```python
from build123d import *

# Parameters (mm, degrees)
BOSS_EXTRU_1_DEPTH      = 26
ESQUISSE2_R             = 12
ENL_V_MAT_EXTRU_1_DEPTH = 27
ESQUISSE3_W             = 35.8
ESQUISSE3_H             = 18
ESQUISSE3_W_2           = 20.2
ESQUISSE3_H_2           = 20.2
ENL_V_MAT_EXTRU_2_DEPTH = 43.5
ESQUISSE4_W             = 15
ESQUISSE4_H             = 20
ENL_V_MAT_EXTRU_3_DEPTH = 38.5
D_GAGEMENT_M31_D        = 3.3
ENL_V_MAT_EXTRU_4_REACH = 48.2
ESQUISSE7_W             = 6
ESQUISSE7_H             = 16
D_GAGEMENT_M41_D        = 4.4
D_GAGEMENT_M41_DEPTH    = 24
ESQUISSE10_W            = 2.2
ESQUISSE10_H            = 24
ENL_V_MAT_EXTRU_5_REACH = 5
ESQUISSE12_W            = 3
ESQUISSE12_H            = 7


with BuildPart() as part:
    # Esquisse1 → Boss.-Extru.1 (new body)
    with BuildSketch(Plane.XY):
        Polygon((0, 0), (0, -42.5), (86, -42.5), (86, -18.5), (71, 0), align=None)
    extrude(amount=BOSS_EXTRU_1_DEPTH)

    # Esquisse2 → Enlèv. mat.-Extru.1 (cut, through all)
    with BuildSketch(Plane.XY.offset(26)):
        with Locations((22, -21.25)):
            Circle(ESQUISSE2_R)
    extrude(amount=-ENL_V_MAT_EXTRU_1_DEPTH, mode=Mode.SUBTRACT)

    # Esquisse3 → Enlèv. mat.-Extru.2 (cut, through all)
    with BuildSketch(Plane(origin=(0, 0, 0), x_dir=(1, 0, 0), z_dir=(0, 1, 0))):
        with Locations((21.9, -13)):
            Rectangle(ESQUISSE3_W, ESQUISSE3_H)
        with Locations((53.9, -13)):
            Rectangle(ESQUISSE3_W_2, ESQUISSE3_H_2)
    extrude(amount=-ENL_V_MAT_EXTRU_2_DEPTH, mode=Mode.SUBTRACT)

    # Esquisse4 → Enlèv. mat.-Extru.3 (cut)
    with BuildSketch(Plane(origin=(0, 0, 0), x_dir=(1, 0, 0), z_dir=(0, 1, 0))):
        with Locations((78.5, -13)):
            Rectangle(ESQUISSE4_W, ESQUISSE4_H)
    extrude(amount=-ENL_V_MAT_EXTRU_3_DEPTH, mode=Mode.SUBTRACT)

    # Dégagement M31 (through all)
    with Locations(Plane.XY.offset(26)):
        with Locations((22, -21.25), (37.5, -36.75), (6.5, -5.75), (6.5, -36.75), (37.5, -5.75)):
            Hole(D_GAGEMENT_M31_D / 2)

    # Esquisse7 → Enlèv. mat.-Extru.4 (cut, up to next)
    with BuildSketch(Plane.ZY.offset(-39.8), mode=Mode.PRIVATE) as enl_v_mat_extru_4_sk1:
        with Locations((13, -8)):
            Rectangle(ESQUISSE7_W, ESQUISSE7_H)
    enl_v_mat_extru_4_tool1 = extrude(enl_v_mat_extru_4_sk1.sketch, amount=-ENL_V_MAT_EXTRU_4_REACH, mode=Mode.PRIVATE) & part.part
    add(enl_v_mat_extru_4_tool1.solids().sort_by_distance((39.8, -8, 13))[0], mode=Mode.SUBTRACT)
    # Esquisse7 → Enlèv. mat.-Extru.4 (cut, up to next)
    with BuildSketch(Plane.ZY.offset(-39.8), mode=Mode.PRIVATE) as enl_v_mat_extru_4_sk2:
        with Locations((13, -34.5)):
            Rectangle(ESQUISSE7_W, ESQUISSE7_H)
    enl_v_mat_extru_4_tool2 = extrude(enl_v_mat_extru_4_sk2.sketch, amount=-ENL_V_MAT_EXTRU_4_REACH, mode=Mode.PRIVATE) & part.part
    add(enl_v_mat_extru_4_tool2.solids().sort_by_distance((39.8, -34.5, 13))[0], mode=Mode.SUBTRACT)

    # Dégagement M41
    with Locations(Plane(origin=(0, -38.5, 0), x_dir=(1, 0, 0), z_dir=(0, 1, 0))):
        with Locations((78, -13)):
            Hole(D_GAGEMENT_M41_D / 2, depth=D_GAGEMENT_M41_DEPTH)

    # Esquisse10 → Dégagement M42 (revolve, cut)
    with BuildSketch(Plane(origin=(78, -28.5, 23), x_dir=(0, 1, 0), z_dir=(1, 0, 0))):
        with Locations((1.1, 12)):
            Rectangle(ESQUISSE10_W, ESQUISSE10_H)
    revolve(axis=Axis((78, -28.5, 16.65), (0, 0, 1)), mode=Mode.SUBTRACT)

    # Esquisse12 → Enlèv. mat.-Extru.5 (cut, up to next)
    with BuildSketch(Plane.XY.offset(3), mode=Mode.PRIVATE) as enl_v_mat_extru_5_sk1:
        with Locations((78.5, -28.5)):
            Rectangle(ESQUISSE12_W, ESQUISSE12_H)
    enl_v_mat_extru_5_tool1 = extrude(enl_v_mat_extru_5_sk1.sketch, amount=-ENL_V_MAT_EXTRU_5_REACH, mode=Mode.PRIVATE) & part.part
    add(enl_v_mat_extru_5_tool1.solids().sort_by_distance((78.5, -28.5, 3))[0], mode=Mode.SUBTRACT)


solid = part.part
```
Design review of the part built by this model. Coordinates are the model's own, in mm. A direction names the side the tool comes from. Coordinates: 2 decimals unless noted, no trailing zeros. Order: outer loops, then holes, each group sorted by start corner. A loop starts at its lowest first (then second) coordinate and runs counter-clockwise, first axis right, second up. Notation, with made-up numbers: (-1, 23) - (46, 23) arc R24 ccw to (46, 54) - close; hole circle Ø1 at (9.5, -22). An arc over 180 degrees is marked (long way). One line per question, with ' | ' between items.
Q1. Consider section B-B, the plane x = 37.5. Give the boundary of the cut face in (y, z).
Answer key:
outline: (-42.5, 0) - (-38.4, 0) - (-38.4, 4) - (-42.5, 4) - close; (-42.5, 22) - (-38.4, 22) - (-38.4, 26) - (-42.5, 26) - close; (-35.1, 0) - (-7.4, 0) - (-7.4, 4) - (-35.1, 4) - close; (-35.1, 22) - (-7.4, 22) - (-7.4, 26) - (-35.1, 26) - close; (-4.1, 0) - (0, 0) - (0, 4) - (-4.1, 4) - close; (-4.1, 22) - (0, 22) - (0, 26) - (-4.1, 26) - close
Q2. Clearance check with flat-ended pins moving along their axes: pin 1 Ø7.5 at (x, z) = (79.5, 9.5) entering from +Y; pin 2 Ø8 at (y, z) = (-13.5, 20) entering from +X; pin 3 Ø1.5 at (y, z) = (-24, 11.5) entering from +X. State where each tip first meets the part, or that it passes through.
Answer key:
pin 1: stops at y = -38.5 | pin 2: stops at x = 84.09 | pin 3: stops at x = 71
Q3. For faces 4 (the flat face through (77, -29, 2)), 5 (the cylindrical face through (20.44, -9.35, 24.03)), 6 (the flat face through (78.4, -38.5, 10.6)), 7 (the flat face through (9.7, -21, 22)), list the 3-axis set-ups (+Z, -Z, +X, -X, +Y, -Y) from which the entire face can be reached by the end or side of a thin tool; tool diameter is ignored.
Answer key:
face 4: -Z | face 5: +Z, -Z | face 6: +X, +Y | face 7: +Y, -Y
Q4. Consider section A-A, the plane y = -21.25. Give the boundary of the cut face in (x, z), then the cut area to 3 significant figures.
Answer key:
outline: (0, 0) - (10, 0) - (10, 4) - (4, 4) - (4, 22) - (10, 22) - (10, 26) - (0, 26) - close; (34, 0) - (86, 0) - (86, 3) - (71, 3) - (71, 23) - (86, 23) - (86, 26) - (34, 26) - (34, 22) - (39.8, 22) - (39.8, 4) - (34, 4) - close; hole (43.8, 2.9) - (64, 2.9) - (64, 23.1) - (43.8, 23.1) - close | area: 692 mm2
Q5. Consider section D-D, the plane z = 2. Give the boundary of the cut face in (x, y), then the cut area to 3 significant figures.
Answer key:
outline: (0, -42.5) - (86, -42.5) - (86, -18.5) - (71, 0) - (0, 0) - close; hole circle Ø3.3 at (6.5, -36.75); hole circle Ø3.3 at (6.5, -5.75); hole circle Ø24 at (22, -21.25); hole circle Ø3.3 at (37.5, -36.75); hole circle Ø3.3 at (37.5, -5.75); hole (77, -32) - (80, -32) - (80, -25) - (77, -25) - close | area: 3,010 mm2
Q6. Consider section C-C, the plane z = 13. Give the boundary of the cut face in (x, y).
Answer key:
outline: (0, -42.5) - (4, -42.5) - (4, 0) - (0, 0) - close; (39.8, -26.5) - (43.8, -26.5) - (43.8, -16) - (39.8, -16) - close; (64, -42.5) - (75.8, -42.5) - (75.8, -38.5) - (71, -38.5) - (71, 0) - (64, 0) - close; (80.2, -42.5) - (86, -42.5) - (86, -38.5) - (80.2, -38.5) - close
Q7. The part is to be moulded in two halves that separate along X. For faces 1 (the flat face through (86, -39, 13)), 2 (the flat face through (0, -21, 13)), 3 (the flat face through (42, -8, 10)), say which applies: +X half, -X half, draft (parallel to the pull), parting line (faces both ways), or undercut.
Answer key:
face 1: +X half | face 2: -X half | face 3: undercut
Q8. To check wall thickness, follow line 1 along Y through (x, z) = (37.5, 24.5); line 2 along X through (y, z) = (-20, 9.75); line 3 along X through (y, z) = (-39, 7). State the ranges of each line that lie inside material, in increasing order.
Answer key:
line 1: y = -42.5 to -38.4, -35.1 to -7.4, -4.1 to 0 | line 2: x = 0 to 4, 39.8 to 43.8, 64 to 71 | line 3: x = 0 to 4, 39.8 to 43.8, 64 to 86
